from build123d import *

# Parameters (mm, degrees)
SKETCH1_W           = 50.8
SKETCH1_H           = 50.8
SKETCH1_R           = 2.5527
SKETCH1_W_2         = 63.5
SKETCH1_H_2         = 25.4
BOSS_EXTRUDE1_DEPTH = 4.7625


with BuildPart() as part:
    # Sketch1 → Boss-Extrude1 (new body)
    # profile 1 of 2: a face of its own
    with BuildSketch(Plane.XY):
        with Locations((25.4, 25.4)):
            Rectangle(SKETCH1_W, SKETCH1_H)
        with Locations(Location((38.1, 12.7, 0), (0, 0, 180))):
            Circle(SKETCH1_R, mode=Mode.SUBTRACT)
        with Locations(Location((12.7, 12.7, 0), (0, 0, 180))):
            Circle(SKETCH1_R, mode=Mode.SUBTRACT)
    # profile 2 of 2: a face of its own
    with BuildSketch(Plane.XY):
        with Locations((-31.75, 38.1)):
            Rectangle(SKETCH1_W_2, SKETCH1_H_2)
        with Locations(Location((-55.88, 38.1, 0), (0, 0, 180))):
            Circle(SKETCH1_R, mode=Mode.SUBTRACT)
    extrude(amount=BOSS_EXTRUDE1_DEPTH)


solid = part.part
Input: part model. Units: mm. Frame: model coordinates. A direction names the side the tool comes from. Coordinates: 2 decimals unless noted, no trailing zeros. Order: outer loops, then holes, each group sorted by start corner. A loop starts at its lowest first (then second) coordinate and runs counter-clockwise, first axis right, second up.
1. Cut plane D-D, the plane y = 12.7. Return loops of the section in (x, z).
Checked values:
outline: (0, 0) - (10.15, 0) - (10.15, 4.76) - (0, 4.76) - close; (15.25, 0) - (35.55, 0) - (35.55, 4.76) - (15.25, 4.76) - close; (40.65, 0) - (50.8, 0) - (50.8, 4.76) - (40.65, 4.76) - close
2. Draft query along Y for faces 3 (the flat face through (50.8, 25, 2)), 4 (the flat face through (25, 0, 2)), 5 (the cylindrical face through (-55.55, 35.57, 2.35)), 6 (the cylindrical face through (10.342, 13.678, 2.348)). Return one class per face: +Y half, -Y half, draft (parallel to the pull), parting line (faces both ways), or undercut.
Checked values:
face 3: draft
face 4: -Y half
face 5: undercut
face 6: undercut
3. Cut plane C-C, the plane z = 2.3. Return loops of the section in (x, y), plus the area to 3 significant figures.
Checked values:
outline: (-63.5, 25.4) - (0, 25.4) - (0, 0) - (50.8, 0) - (50.8, 50.8) - (-63.5, 50.8) - close; hole circle Ø5.11 at (-55.88, 38.1); hole circle Ø5.11 at (12.7, 12.7); hole circle Ø5.11 at (38.1, 12.7)
area: 4,130 mm2
4. Ray query, line 1 along X through (y, z) = (12.7, 1.85); line 2 along X through (y, z) = (38.1, 2.5); line 3 along X through (y, z) = (10.5, 3.2). Return the intervals inside material, ascending.
Checked values:
line 1: x = 0 to 10.15, 15.25 to 35.55, 40.65 to 50.8
line 2: x = -63.5 to -58.43, -53.33 to 50.8
line 3: x = 0 to 11.41, 13.99 to 36.81, 39.39 to 50.8
5. Contact query for flat-ended pins moving along their axis: P1, Ø3, axis at x = 12.7, y = 12.7, coming from the -Z side; P2, Ø2.5, axis at x = -24, z = 3, coming from the -Y side. Output: stop coordinate, or through.
Checked values:
P1: passes through
P2: stops at y = 25.4
6. Access query for faces 1 (the flat face through (0, 13, 2)), 2 (the flat face through (-63.5, 38, 2)). Directions: +Z, -Z, +X, -X, +Y, -Y. A direction counts if a zero-diameter tool reaches every point of the face in a straight line with its end or side. Return the directions, or none.
Checked values:
face 1: +Z, -Z, -X, -Y
face 2: +Z, -Z, -X, +Y, -Y
7. Cut plane A-A, the plane y = 38.1. Return loops of the section in (x, z).
Checked values:
outline: (-63.5, 0) - (-58.43, 0) - (-58.43, 4.76) - (-63.5, 4.76) - close; (-53.33, 0) - (50.8, 0) - (50.8, 4.76) - (-53.33, 4.76) - close
8. Cut plane B-B, the plane x = -55.88. Return loops of the section in (y, z).
Checked values:
outline: (25.4, 0) - (35.55, 0) - (35.55, 4.76) - (25.4, 4.76) - close; (40.65, 0) - (50.8, 0) - (50.8, 4.76) - (40.65, 4.76) - close
